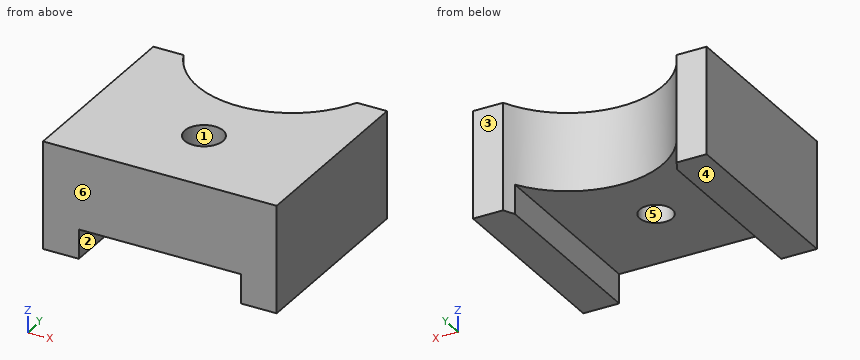
Autodesk Inventor part; units mm, degrees
ref_plane "YZ Plane" through (0, 0, 0) normal (1, 0, 0) x (0, 1, 0)
ref_plane "XZ Plane" through (0, 0, 0) normal (0, 1, 0) x (-1, 0, 0)
ref_plane "XY Plane" through (0, 0, 0) normal (0, 0, 1) x (1, 0, 0)
sketch "Sketch3" plane through (0, 0, 0) normal (0, 0, 1) x (1, 0, 0)
  line L0 (-12.7, -19.05) -> (12.7, -19.05)
  line L1 (12.7, -19.05) -> (12.7, 19.05)
  line L2 (12.7, 19.05) -> (-12.7, 19.05)
  line L3 (-12.7, 19.05) -> (-12.7, -19.05)
  line L4 (-12.7, -19.05) -> (12.7, 19.05) construction
  line L5 (12.7, -19.05) -> (-12.7, 19.05) construction
  point P0 (0, 0)
  dimension "d0" = 25.4
  dimension "d1" = 38.1
extrude "Extrusion1" add sketch "Sketch3" along normal mid plane 12.7
sketch "Sketch4" plane through (0, 0, 6.35) normal (0, 0, 1) x (1, 0, 0)
  circle A0 centre (0, 0) radius 2.667
  dimension "d4" = 5.334
extrude "Extrusion2" cut sketch "Sketch4" against normal through all
sketch "Sketch5" plane through (-12.7, -19.05, 6.35) normal (-1, 0, 0) x (0, 0, 1)
  line L0 (3.175, 6.35) -> (50.8, 6.35)
  line L1 (-12.7, 38.1) -> (-12.7, 0)
  line L2 (0, 0) -> (0, 38.1)
  line L3 (-12.7, 0) -> (0, 0)
  line L4 (0, 0) -> (0, 6.35)
  line L5 (0, 6.35) -> (-12.7, 6.35)
  line L6 (-12.7, 6.35) -> (-12.7, 0)
  point P0 (-6.35, 19.05)
  point P1 (-12.7, 6.35)
  dimension "d9" = 6.35
extrude "Extrusion3" cut sketch "Sketch5" against normal through all
sketch "Sketch8" plane through (-12.7, -12.7, -6.35) normal (-1, 0, 0) x (0, 0, 1)
  line L0 (-4.7625, 21.8398) -> (-4.7625, 13.2284)
  line L1 (12.7, 0) -> (12.7, 31.75)
  line L2 (12.7, 0) -> (-4.7625, 0)
  line L3 (-4.7625, 0) -> (-4.7625, 31.75)
  line L4 (-4.7625, 31.75) -> (12.7, 31.75)
  line L5 (12.7, 31.75) -> (12.7, 0)
  point P0 (6.35, 12.7)
  point P1 (-4.7625, 13.2284)
extrude "Extrusion5" add sketch "Sketch8" along normal blind 6.35
mirror "Mirror1" about plane through (0, 0, 0) normal (1, 0, 0) of "Extrusion5"
sketch "Sketch6" plane through (0, 0, 0) normal (0, 0, 1) x (1, 0, 0)
  circle A0 centre (0, 25.4) radius 15.494
  point P0 (0, 0)
  dimension "d10" = 25.4
  dimension "d13" = 30.988
extrude "cutOutForGuide" cut sketch "Sketch6" along normal through all both and the other way through all
sketch "Sketch9" plane through (0, 0, 6.35) normal (0, 0, 1) x (1, 0, 0)
  circle A0 centre (0, 0) radius 3.1242
  dimension "d16" = 6.2484
extrude "Extrusion6" cut sketch "Sketch9" against normal blind 9.525
sketch "Sketch10" plane through (-12.7, -12.7, -11.1125) normal (0, 0, -1) x (-1, 0, 0)
  line L0 (0, 0) -> (6.35, 0)
  line L1 (0, 0) -> (0.508, 0)
  line L2 (0.508, 0) -> (0.508, 36.9717)
  line L3 (0.508, 36.9717) -> (0, 36.9717)
  line L4 (0, 36.9717) -> (0, 0)
  point P0 (-12.7, 12.7)
  point P1 (0.508, 0)
  dimension "d19" = 0.508
extrude "Extrusion7" cut sketch "Sketch10" against normal blind 4.7625
mirror "Mirror2" about plane through (0, 0, 0) normal (1, 0, 0) of "Extrusion7"
properties part number "leo" material "PBT Plastic"
Build history of the part. All positions in model axes, mm. Face numbers are marked on the shaded views. A direction names the side the tool comes from. Round coordinates to 2 decimals unless told otherwise and drop trailing zeros. Write each loop counter-clockwise with the first axis right and the second up, starting at its lowest first coordinate (ties: lowest second). Pieces come first, ordered by that corner, then holes. Notation, with made-up numbers: (18, 9.25) - (68, 9.25) arc R29 ccw to (68, 40.25) - close; hole circle Ø6 at (-38.75, 11). An arc over 180 degrees is marked (long way). One line per question, with ' | ' between items.
1. Band-saw the part on D-D, the plane z = 4. Write the cut outline in (x, y), and give its area (3 significant figures).
Results are:
outline: (-19.05, -12.7) - (19.05, -12.7) - (19.05, 19.05) - (14.13, 19.05) arc R15.49 cw to (-14.13, 19.05) - (-19.05, 19.05) - close; hole circle Ø6.25 at (0, 0) | area: 993 mm^2
2. Mould opens along Y. For the marked faces 4, 5 and 6 say: released by +Y, released by -Y, zero draft, split by the parting line, or undercut.
Results are:
face 4: zero draft | face 5: undercut | face 6: released by -Y
3. Tool access for the marked faces 1, 2 and 3: list every direction of +Z, -Z, +X, -X, +Y, -Y with a clear straight run to the whole face (end or side of a thin tool).
Results are:
face 1: +Z | face 2: -Z, +Y, -Y | face 3: +Z, -Z, +X, -X, +Y
4. Band-saw the part on C-C, the plane x = 0. Write the cut outline in (y, z) (3 decimals), and give its area (3 significant figures).
Results are:
outline: (-12.7, -6.35) - (-2.667, -6.35) - (-2.667, -3.175) - (-3.124, -3.175) - (-3.124, 6.35) - (-12.7, 6.35) - close; (2.667, -6.35) - (9.906, -6.35) - (9.906, 6.35) - (3.124, 6.35) - (3.124, -3.175) - (2.667, -3.175) - close | area: 211 mm^2
5. Drop flat-ended pins along their axis: pin 1 Ø5.5 at (x, y) = (0, 0) entering from +Z (3 decimals); pin 2 Ø8.5 at (x, y) = (0, 0) entering from -Z; pin 3 Ø10 at (x, z) = (-5, -4) entering from +Y. Give the stop position or say it passes through.
Results are:
pin 1: z = -3.175 | pin 2: z = -6.35 | pin 3: y = 13.57
6. Drill centre lines: line 1 along Y through (x, z) = (0, 3.5); line 2 along Y through (x, z) = (0, -4); line 3 along Z through (x, y) = (-6, -5.5). Where is each one in solid material? Low to high. Write a range as from..to.
Results are:
line 1: -12.7..-3.12, 3.12..9.91 | line 2: -12.7..-2.67, 2.67..9.91 | line 3: -6.35..6.35
7. Band-saw the part on A-A, the plane z = -9. Write the cut outline in (x, y), and give its area (3 significant figures).
Results are:
outline: (-19.05, -12.7) - (-13.21, -12.7) - (-13.21, 17.3) arc R15.49 cw to (-14.13, 19.05) - (-19.05, 19.05) - close; (13.21, -12.7) - (19.05, -12.7) - (19.05, 19.05) - (14.13, 19.05) arc R15.49 cw to (13.21, 17.3) - close | area: 369 mm^2
